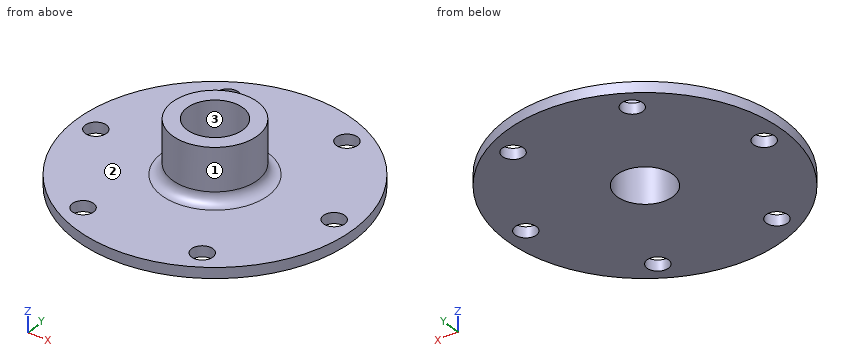
from build123d import *

# Parameters (mm, degrees)
SKETCH2_R          = 8.324772978
CUT_EXTRUDE5_DEPTH = 62.401577748
SKETCH3_R          = 3.175
CUT_EXTRUDE6_DEPTH = 61.491874454
CIRPATTERN2_COUNT  = 6
FILLET1_R          = 3.175


with BuildPart() as part:
    # Sketch1 → Revolve1 (revolve)
    with BuildSketch(Plane(origin=(0, 0, 0), x_dir=(0, 0, -1), z_dir=(1, 0, 0)), mode=Mode.PRIVATE) as revolve1_sk:
        Polygon((0, 0), (0, 41.275), (-3.175, 41.275), (-3.175, 12.7), (-19.05, 12.7), (-19.05, 0), align=None)
    revolve(revolve1_sk.sketch.rotate(Axis((0, 0, 0), (0, 0, 1)), 90), axis=Axis((0, 0, 0), (0, 0, 1)))

    # Sketch2 → Cut-Extrude5 (cut, through all)
    with BuildSketch(Plane.XY):
        with Locations(Location((0, 0, 0), (0, 0, 180))):
            Circle(SKETCH2_R)
    extrude(amount=CUT_EXTRUDE5_DEPTH, mode=Mode.SUBTRACT)

    # Sketch3 → Cut-Extrude6 (cut, through all)
    with BuildSketch(Plane.XY.offset(3.175)):
        with Locations((34.925, 0)):
            Circle(SKETCH3_R)
    cut_extrude6 = extrude(amount=-CUT_EXTRUDE6_DEPTH, mode=Mode.SUBTRACT)

    # CirPattern2: Cut-Extrude6 ×6 about axis
    cirpattern2_axis = Axis((0, 0, 0), (0, 0, 1))
    for i in range(1, CIRPATTERN2_COUNT):
        add(cut_extrude6.rotate(cirpattern2_axis, i * 360 / CIRPATTERN2_COUNT), mode=Mode.SUBTRACT)

    # Fillet1
    fillet1_edges = [part.edges().sort_by_distance(p)[0] for p in [
        (12.7, 0, 3.175),
    ]]
    fillet(fillet1_edges, radius=FILLET1_R)


solid = part.part
CAD build for the part. Positions are in the model's coordinates, mm. Face numbers are marked on the shaded views. Give positions to 0.01 mm unless a question says otherwise; leave off trailing zeros. Loops run counter-clockwise (first coordinate to the right, second up) from the corner with the lowest first, then second, coordinate; pieces in that order, holes last. Notation, with made-up numbers: M 80,37.25 L 85,37.25 A15 ccw 85,53.25 Z; hole C -38.75,-31.5 d7. An arc over 180 degrees is marked long. Answer in a Markdown table with one row per item. Add a question column.
Item 1: Band-saw the part on B-B on y = 0. Give the cut face in (x, z) (3 decimals), then the cut area to 3 significant figures.
Item 2: Band-saw the part on A-A on x = 0. Give the cut face in (y, z) (3 decimals).
Item 3: Probe probe 1 along Y at (x, z) = (0, 12.5); probe 2 along Z at (x, y) = (-32, 5.5) (3 decimals); probe 3 along X at (y, z) = (6, 5.5). List the from-to ranges inside material, lowest first.
Item 4: Band-saw the part on C-C on z = 10.25. Give the cut face in (x, y), then the cut area to 3 significant figures.
Item 5: Band-saw the part on D-D on y = 18. Give the cut face in (x, z) (3 decimals), then the cut area to 3 significant figures.
Item 6: Drop flat-ended pins along their axis: P1, Ø8.5, axis at x = -17.46, y = -30.25, coming from the +Z side (3 decimals); P2, Ø6, axis at y = -18.5, z = 7, coming from the -X side; P3, Ø10, axis at x = -8.5, z = 11, coming from the -Y side; P4, Ø6, axis at x = 13, z = 15, coming from the -Y side. Give the stop position or say it passes through.
Item 7: Mould opens along X. For the marked faces 1, 2 and 3 say: +X half, -X half, draft (parallel to the pull), parting line (faces both ways), or undercut.
Reply:
| question | item | result |
|---|---|---|
| 1 | outline | M -41.275,0 L -38.1,0 L -38.1,3.175 L -41.275,3.175 Z; M -31.75,0 L -8.325,0 L -8.325,19.05 L -12.7,19.05 L -12.7,6.35 A3.175 cw -15.875,3.175 L -31.75,3.175 Z; M 8.325,0 L 31.75,0 L 31.75,3.175 L 15.875,3.175 A3.175 cw 12.7,6.35 L 12.7,19.05 L 8.325,19.05 Z; M 38.1,0 L 41.275,0 L 41.275,3.175 L 38.1,3.175 Z |
| 1 | area | 312 mm^2 |
| 2 | outline | M -41.275,0 L -8.325,0 L -8.325,19.05 L -12.7,19.05 L -12.7,6.35 A3.175 cw -15.875,3.175 L -41.275,3.175 Z; M 8.325,0 L 41.275,0 L 41.275,3.175 L 15.875,3.175 A3.175 cw 12.7,6.35 L 12.7,19.05 L 8.325,19.05 Z |
| 3 | probe 1 | y = -12.7 to -8.32, 8.32 to 12.7 |
| 3 | probe 2 | z = 0 to 3.175 |
| 3 | probe 3 | x = -11.32 to -5.77, 5.77 to 11.32 |
| 4 | outline | C 0,0 d25.4; hole C 0,0 d16.65 |
| 4 | area | 289 mm^2 |
| 5 | outline | M -37.143,0 L 37.143,0 L 37.143,3.175 L -37.143,3.175 Z |
| 5 | area | 236 mm^2 |
| 6 | P1 | stops at z = 3.175 |
| 6 | P2 | passes through |
| 6 | P3 | stops at y = -12.21 |
| 6 | P4 | stops at y = -7.83 |
| 7 | face 1 | parting line |
| 7 | face 2 | draft |
| 7 | face 3 | undercut |
